from build123d import *

# Parameters (mm, degrees)
PAD018_DEPTH = 1.92
SKETCH042_W  = 28
SKETCH042_H  = 26
SKETCH042_R  = 2
PAD020_DEPTH = 6
PAD021_DEPTH = 2.4


with BuildPart() as part:
    # Sketch038 → Pad018 (new body)
    with BuildSketch(Plane.XY):
        with BuildLine():
            ThreePointArc((16, -52.6212884677), (54.5217663163, -7.237195434), (29.1738989847, 46.6249248582))
            ThreePointArc((28, 48.7442306082), (28.3130783141, 47.5328784807), (29.1738989848, 46.6249248582))
            Line((28, 52.3787115323), (28, 48.7442306082))
            Line((0, 52.3787115323), (28, 52.3787115323))
            Line((0, 46.3787115323), (0, 52.3787115323))
            Line((13.5000003539, 46.3787115323), (0, 46.3787115323))
            ThreePointArc((16, 43.8787114546), (15.2677671056, 45.6464783327), (13.5000003539, 46.3787115323))
            Line((16, 43.8787114546), (16, -52.6212884677))
        make_face()
    pad018 = extrude(amount=PAD018_DEPTH)

    # Sketch042 (on DatumPlane) → Pad020 (join)
    with BuildSketch(Plane(origin=(0, 52.3787115323, 0), x_dir=(-1, 0, 0), z_dir=(0, 1, 0))):
        with Locations((-14, 13)):
            Rectangle(SKETCH042_W, SKETCH042_H)
        with Locations((-13, 13)):
            Circle(SKETCH042_R, mode=Mode.SUBTRACT)
    pad020 = extrude(amount=-PAD020_DEPTH)

    # Sketch043 (on DatumPlane) → Pad021 (join)
    with BuildSketch(Plane(origin=(23, 0, 0), x_dir=(0, -1, 0), z_dir=(-1, 0, 0))):
        Polygon((-46.3787115323, 26), (48.344858, 1.92), (-46.3787115323, 1.92), align=None)
    pad021 = extrude(amount=PAD021_DEPTH)

    # Mirrored011: Pad018, Pad020, Pad021 across Sketch038 V_Axis
    add(pad018.mirror(Plane(origin=(0, 0, 0), x_dir=(0, 0, 1), z_dir=(1, 0, 0))))
    add(pad020.mirror(Plane(origin=(0, 0, 0), x_dir=(0, 0, 1), z_dir=(1, 0, 0))))
    add(pad021.mirror(Plane(origin=(0, 0, 0), x_dir=(0, 0, 1), z_dir=(1, 0, 0))))


solid = part.part
Verification items for the finished model (mm, model axes). A direction names the side the tool comes from. Coordinates: 2 decimals unless noted, no trailing zeros. Write each loop counter-clockwise with the first axis right and the second up, starting at its lowest first coordinate (ties: lowest second). Pieces come first, ordered by that corner, then holes. Notation, with made-up numbers: M 23.5,34 L 28.5,34 A24 cw 28.5,65 Z; hole C 37,64.25 d5. An arc over 180 degrees is marked long. Use a Markdown table: item, result.
Q1. Thickness scan on line 1 (X direction, y = 3.5, z = 4.5); line 2 (Z direction, x = 13, y = 47.7); line 3 (Y direction, x = 20, z = 8.5). Record the ranges inside material, lowest first.
Reply:
| item | result |
|---|---|
| line 1 | x = -23 to -20.6, 20.6 to 23 |
| line 2 | z = 0 to 11, 15 to 26 |
| line 3 | y = 46.38 to 52.38 |
Q2. Draft check along X on faces 5 (the face through (23, 19, 9)), 6 (the face through (34, -1, 1.92)), 7 (the face through (-21.82, -0.32, 14.13)), 8 (the face through (-34, -1, 1.92)). Enter one of: +X half, -X half, draft (parallel to the pull), parting line (faces both ways), or undercut.
Reply:
| item | result |
|---|---|
| face 5 | +X half |
| face 6 | undercut |
| face 7 | draft |
| face 8 | undercut |
Q3. Sectioned sample at B-B, the plane z = 13. Record the boundary of the cut face in (x, y), plus the area to 3 significant figures.
Reply:
| item | result |
|---|---|
| outline | M -28,46.38 L -23,46.38 L -23,-4.76 L -20.6,-4.76 L -20.6,46.38 L -15,46.38 L -15,52.38 L -28,52.38 Z; M -11,46.38 L 11,46.38 L 11,52.38 L -11,52.38 Z; M 15,46.38 L 20.6,46.38 L 20.6,-4.76 L 23,-4.76 L 23,46.38 L 28,46.38 L 28,52.38 L 15,52.38 Z |
| area | 533 mm² |
Q4. Sectioned sample at C-C, the plane y = -25.5. Record the boundary of the cut face in (x, z).
Reply:
| item | result |
|---|---|
| outline | M -48.73,0 L -16,0 L -16,1.92 L -20.6,1.92 L -20.6,7.73 L -23,7.73 L -23,1.92 L -48.73,1.92 Z; M 16,0 L 48.73,0 L 48.73,1.92 L 23,1.92 L 23,7.73 L 20.6,7.73 L 20.6,1.92 L 16,1.92 Z |
Q5. Set-up check for faces 1 (the face through (26, 46.379, 14)), 2 (the face through (-15.287, 45.627, 0.947)), 3 (the face through (20.6, 19, 9)), 4 (the face through (-26, 46.379, 14)): record each of +Z, -Z, +X, -X, +Y, -Y from which the full face is reachable in a straight line by a thin tool's end or side.
Reply:
| item | result |
|---|---|
| face 1 | +Z, +X, -Y |
| face 2 | +Z, -Z, -Y |
| face 3 | +Z, -Y |
| face 4 | +Z, -X, -Y |
Q6. Sectioned sample at A-A, the plane y = 41.5. Record the boundary of the cut face in (x, z).
Reply:
| item | result |
|---|---|
| outline | M -36.09,0 L -16,0 L -16,1.92 L -20.6,1.92 L -20.6,24.76 L -23,24.76 L -23,1.92 L -36.09,1.92 Z; M 16,0 L 36.09,0 L 36.09,1.92 L 23,1.92 L 23,24.76 L 20.6,24.76 L 20.6,1.92 L 16,1.92 Z |
Q7. Sectioned sample at D-D, the plane z = 24.5. Record the boundary of the cut face in (x, y).
Reply:
| item | result |
|---|---|
| outline | M -28,46.38 L -23,46.38 L -23,40.48 L -20.6,40.48 L -20.6,46.38 L 20.6,46.38 L 20.6,40.48 L 23,40.48 L 23,46.38 L 28,46.38 L 28,52.38 L -28,52.38 Z |
Q8. Go/stop test with flat-tipped pins: P1, Ø12, axis at y = -17, z = 12.5, coming from the -X side; P2, Ø4.5, axis at x = -13, z = 13, coming from the +Y side; P3, Ø12, axis at x = 25.5, z = 4, coming from the -Y side; P4, Ø1.5, axis at y = -25, z = 1, coming from the -X side. Record where each tip stops, or that it passes through.
Reply:
| item | result |
|---|---|
| P1 | stops at x = -23 |
| P2 | stops at y = 52.38 |
| P3 | stops at y = -51.28 |
| P4 | stops at x = -49.37 |
